```python
from build123d import *

# Parameters (mm, degrees)
SKETCH1_W                    = 146.05
SKETCH1_H                    = 76.2
BOSS_EXTRUDE1_DEPTH          = 3.175
F_1_8_0_125_DIAMETER_HOLE1_D = 3.175
F_1_2_0_5_DIAMETER_HOLE1_D   = 12.7
F_6_CLEARANCE_HOLE1_D        = 4.3053
F_4_CLEARANCE_HOLE1_D        = 3.4544


with BuildPart() as part:
    # Sketch1 → Boss-Extrude1 (new body)
    with BuildSketch(Plane.XY):
        with Locations((-73.025, 38.1)):
            Rectangle(SKETCH1_W, SKETCH1_H)
    extrude(amount=-BOSS_EXTRUDE1_DEPTH)

    # 1/8 (0.125) Diameter Hole1 (through all)
    with Locations(Plane(origin=(0, 0, -3.175), x_dir=(-1, 0, 0), z_dir=(0, 0, -1))):
        with Locations((95.25, 55.118), (119.0625, 18.923), (62.23, 55.118), (33.3375, 38.227)):
            Hole(F_1_8_0_125_DIAMETER_HOLE1_D / 2)

    # 1/2 (0.5) Diameter Hole1 (through all)
    with Locations(Plane(origin=(0, 0, -3.175), x_dir=(-1, 0, 0), z_dir=(0, 0, -1))):
        with Locations((95.25, 45.466), (119.0625, 28.575), (62.23, 45.466), (33.3375, 28.575)):
            Hole(F_1_2_0_5_DIAMETER_HOLE1_D / 2)

    # #6 Clearance Hole1 (through all)
    with Locations(Plane(origin=(0, 0, -3.175), x_dir=(-1, 0, 0), z_dir=(0, 0, -1))):
        with Locations((141.1605, 61.9125), (141.1605, 14.2875), (4.8895, 61.9125), (4.8895, 14.2875), (111.125, 66.04), (100.01504, 10.16), (34.925, 66.04)):
            Hole(F_6_CLEARANCE_HOLE1_D / 2)

    # #4 Clearance Hole1 (through all)
    with Locations(Plane(origin=(0, 0, -3.175), x_dir=(-1, 0, 0), z_dir=(0, 0, -1))):
        with Locations((33.3375, 43.18), (33.3375, 13.97)):
            Hole(F_4_CLEARANCE_HOLE1_D / 2)


solid = part.part
```
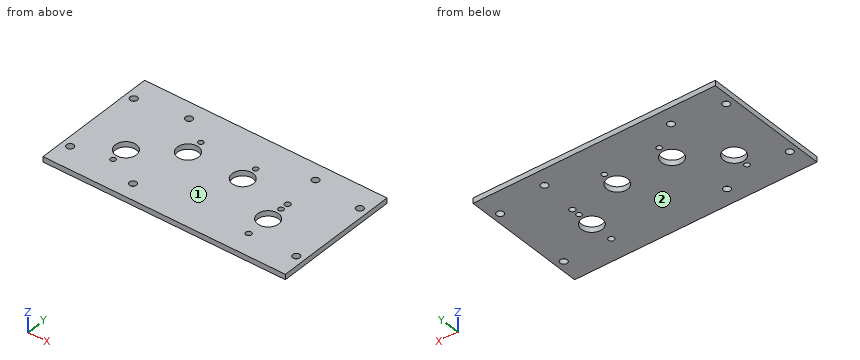
Could you check a few things on this model? Use its own coordinates, in mm. Face numbers are marked on the shaded views. Give positions to 0.01 mm unless a question says otherwise; leave off trailing zeros. Loops run counter-clockwise (first coordinate to the right, second up) from the corner with the lowest first, then second, coordinate; pieces in that order, holes last. Notation, with made-up numbers: (69, -9) -> (94, -9) arc R10 cw to (94, -2) -> close; hole circle Ø10 at (36, -21.75). An arc over 180 degrees is marked (long way). Put each result on its own line as item: value.
(1) I'm going to push a flat-ended pin straight in: pin 1 Ø2.5 at (x, y) = (-4.89, 61.91) entering from -Z. Where does the tip first touch, or does it pass through?
Computed:
pin 1: through
(2) Thinking about a two-plate mould opening in Z: for the marked faces 1 and 2, which applies, pulls with the +Z half, pulls with the -Z half, needs draft (parallel to the pull), parting line crosses it, or undercut?
Computed:
face 1: pulls with the +Z half
face 2: pulls with the -Z half
(3) Imagine slicing it at D-D on z = -2. State how many separate pieces and enclosed holes the cut face has, plus the area to 3 significant figures.
Computed:
separate pieces: 1
enclosed holes: 17
area: 10,500 mm^2
(4) Please list where these lines run through material, in increasing order: probe 1 along Y at (x, z) = (-62.23, -2); probe 2 along X at (y, z) = (62, -2.55); probe 3 along X at (y, z) = (38, -2.35). Write a range as [from, to].
Computed:
probe 1: [0, 39.12], [51.82, 53.53], [56.71, 76.2]
probe 2: [-146.05, -143.31], [-139.01, -7.04], [-2.74, 0]
probe 3: [-146.05, -34.91], [-31.77, 0]
(5) Imagine slicing it at A-A on y = 10.16. Write out the boundary of the cut face in (x, z) (3 decimals).
Computed:
outline: (-146.05, -3.175) -> (-102.168, -3.175) -> (-102.168, 0) -> (-146.05, 0) -> close; (-97.862, -3.175) -> (0, -3.175) -> (0, 0) -> (-97.862, 0) -> close
(6) Imagine slicing it at C-C on y = 49.5. Write out the boundary of the cut face in (x, z) (3 decimals), plus the area to 3 significant figures.
Computed:
outline: (-146.05, -3.175) -> (-100.154, -3.175) -> (-100.154, 0) -> (-146.05, 0) -> close; (-90.346, -3.175) -> (-67.134, -3.175) -> (-67.134, 0) -> (-90.346, 0) -> close; (-57.326, -3.175) -> (0, -3.175) -> (0, 0) -> (-57.326, 0) -> close
area: 401 mm^2
(7) Imagine slicing it at B-B on x = -62.23. Write out the boundary of the cut face in (y, z) (1 decimal), plus the area to 3 significant figures.
Computed:
outline: (0, -3.2) -> (39.1, -3.2) -> (39.1, 0) -> (0, 0) -> close; (51.8, -3.2) -> (53.5, -3.2) -> (53.5, 0) -> (51.8, 0) -> close; (56.7, -3.2) -> (76.2, -3.2) -> (76.2, 0) -> (56.7, 0) -> close
area: 192 mm^2
